Input: part model. Units: mm. Frame: model coordinates. A direction names the side the tool comes from. Coordinates: 2 decimals unless noted, no trailing zeros. Order: outer loops, then holes, each group sorted by start corner. A loop starts at its lowest first (then second) coordinate and runs counter-clockwise, first axis right, second up.
from build123d import *

# Parameters (mm, degrees)
F0_R      = 76.2
F1_DEPTH  = 25.4
F2_R      = 5.08
F3_R      = 19.05
F4_DEPTH  = 12.7
F5_R      = 5.08
F6_R      = 6.35
F7_DEPTH  = 76.2
F8_R      = 7.8213855598
F10_R     = 19.05
F12_DEPTH = 3.81
F13_R     = 7.8169730868
F14_DEPTH = 6.35
F17_DEPTH = 6.35
F19_DEPTH = 8.89
F21_DEPTH = 6.35
F23_DEPTH = 3.81
F25_DEPTH = 3.81


with BuildPart() as f1:
    # F0 (on Front) → F1 (new body)
    with BuildSketch(Plane.XZ):
        Circle(F0_R)
    extrude(amount=F1_DEPTH)

    # F2
    f2_edges = [f1.edges().sort_by_distance(p)[0] for p in [
        (-76.2, 0, 0),
        (-76.2, -25.4, 0),
    ]]
    fillet(f2_edges, radius=F2_R)

    # F3 (on face) → F4 (join)
    with BuildSketch(Plane.XZ.offset(25.4)):
        Circle(F3_R)
    extrude(amount=F4_DEPTH)

    # F5
    f5_edges = [f1.edges().sort_by_distance(p)[0] for p in [
        (-19.05, -38.1, 0),
    ]]
    fillet(f5_edges, radius=F5_R)

    # F6 (on face) → F7 (cut)
    with BuildSketch(Plane.XZ.offset(38.1)):
        Circle(F6_R)
    extrude(amount=-F7_DEPTH, mode=Mode.SUBTRACT)

    # F8 (on Right) → F9 (revolve, cut)
    with BuildSketch(Plane.YZ):
        with Locations((-12.6901438412, 78.25367953)):
            Circle(F8_R)
    revolve(axis=Axis((0, -25.4, 0), (0, -1, 0)), mode=Mode.SUBTRACT)

    # F10 (on face) → F12 (join)
    with BuildSketch(Plane.XZ.offset(25.4)):
        Polygon((47.0374568453, 52.0669616734), (-21.5725830844, 66.7691133941), (-68.6100399297, 14.7021517208), (-47.0374568453, -52.0669616734), (21.5725830844, -66.7691133941), (68.6100399297, -14.7021517208), align=None)
        Circle(F10_R, mode=Mode.SUBTRACT)
    extrude(amount=F12_DEPTH)

    # F13 (on face) → F14 (cut)
    with BuildSketch(Plane.XZ.offset(29.21)):
        with Locations((-25.8648959284, -14.9331046268)):
            Circle(F13_R)
        with Locations((25.8648959284, -14.9331046268)):
            Circle(F13_R)
        with Locations((0, 29.8662092537)):
            Circle(F13_R)
    extrude(amount=-F14_DEPTH, mode=Mode.SUBTRACT)

    # F15 (on face) + F16 (on face) → F17 (cut)
    with BuildSketch(Plane.XZ.offset(29.21)):
        Polygon((-6.4650705634, 63.5317892149), (-14.4013282363, 65.2324158946), (-66.3552315782, 7.7233140955), (-63.8598886488, 0), align=None)
    with BuildSketch(Plane.XZ.offset(29.21)):
        Polygon((0, 61.7343336344), (-61.7343373597, -6.4756297506), (-58.56847018, -14.8219969124), (8.2024643198, 60.0075013936), align=None)
    extrude(amount=-F17_DEPTH, mode=Mode.SUBTRACT)

    # F18 (on face) → F19 (cut)
    with BuildSketch(Plane.XZ.offset(29.21)):
        Polygon((-5.4865229519, 55.6723016167), (-12.2550597484, 57.1227023891), (-16.8224318034, 52.0669616734), (-10.0461006354, 50.6344468321), align=None)
        Polygon((49.692894259, 43.8481405387), (2.757754124, 53.9056707778), (-1.7298993235, 48.8764037987), (51.7189443483, 37.5773306116), align=None)
    extrude(amount=-F19_DEPTH, mode=Mode.SUBTRACT)

    # F20 (on face) → F21 (cut)
    with BuildSketch(Plane.XZ.offset(29.21)):
        Polygon((-24.2682661942, 54.3104504028), (-20.0674166684, 58.960477975), (-27.1381742899, 60.6084184199), (-31.3737366627, 55.9199663113), align=None)
    extrude(amount=-F21_DEPTH, mode=Mode.SUBTRACT)

    # F22 (on face) → F23 (cut)
    with BuildSketch(Plane.XZ.offset(29.21)):
        Polygon((38.5287505055, 40.3657345385), (31.5674540827, 41.8373509918), (57.3507397373, -27.1653585118), (61.4382083927, -22.6408351193), align=None)
    extrude(amount=-F23_DEPTH, mode=Mode.SUBTRACT)

    # F24 (on face) → F25 (cut)
    with BuildSketch(Plane.XZ.offset(29.21)):
        Polygon((29.7542170904, 48.120714307), (36.6590147413, 46.6411147795), (34.266757864, 54.8035400837), (27.7146135315, 56.2075710414), align=None)
    extrude(amount=-F25_DEPTH, mode=Mode.SUBTRACT)


solid = f1.part
Item 1: Ray query, probe 1 along Z at (x, y) = (3.5, -26); probe 2 along Z at (x, y) = (0, -23); probe 3 along Z at (x, y) = (0, -27). Return the intervals inside material, ascending.
Response values:
probe 1: z = -62.9 to -5.3, 5.3 to 22.88, 36.86 to 47.77, 53.75 to 54.74, 61 to 61.4
probe 2: z = -75.44 to -6.35, 6.35 to 22.05, 37.68 to 48.51, 61.73 to 75.44
probe 3: z = -62.15 to -6.35, 6.35 to 22.05, 37.68 to 48.51, 61.73 to 62.15
Item 2: Cut plane A-A on y = -17. Return loops of the section in (x, z), then the cut area to 3 significant figures.
Response values:
outline: circle Ø143.45 at (0, 0); hole circle Ø12.7 at (0, 0)
area: 16,000 mm2
Item 3: Draft query along Z for faces 1 (the face through (-13.213, -27.278, -59.315)), 2 (the face through (-23.553, -26.079, 59.773)), 3 (the face through (-49.73, -27.28, 35.6)). Return one class per face: pulls with the +Z half, pulls with the -Z half, needs draft (parallel to the pull), parting line crosses it, or undercut.
Response values:
face 1: pulls with the -Z half
face 2: undercut
face 3: pulls with the +Z half
Item 4: Access query for faces 4 (the face through (13, -29.21, 56)), 5 (the face through (40.742, -27.278, 53.416)), 6 (the face through (-30, -22.86, 24)), 7 (the face through (-55.566, -27.278, -25.669)). Directions: +Z, -Z, +X, -X, +Y, -Y. A direction counts if a zero-diameter tool reaches every point of the face in a straight line with its end or side. Return the directions, or none.
Response values:
face 4: +Z, +X, -X, -Y
face 5: +Z, +X, -Y
face 6: -Y
face 7: -Z, -X, -Y
Item 5: Pin query (flat end, axial travel): pin 1 Ø9 at (x, z) = (59.5, 10.5) entering from -Y; pin 2 Ø12.5 at (x, z) = (-26.5, -14.5) entering from -Y; pin 3 Ø1.9 at (x, z) = (-12.5, 55) entering from -Y. Return the tip coordinate at first contact, or that it passes through.
Response values:
pin 1: stops at y = -29.21
pin 2: stops at y = -22.86
pin 3: stops at y = -20.32
